Geometry: see drawing. Coordinates: mm, zero at the bounding-box minimum. A direction names the side the tool comes from. Give positions to 0.01 mm unless a question says otherwise; leave off trailing zeros. Order: outer loops, then holes, each group sorted by start corner. A loop starts at its lowest first (then second) coordinate and runs counter-clockwise, first axis right, second up. Notation, with made-up numbers: (82, 51) - (137, 51) arc R30 ccw to (137, 84) - close; hole circle Ø2 at (31.25, -20.5). An arc over 180 degrees is marked (long way). Write item = value, one per line. Start each with the question number.
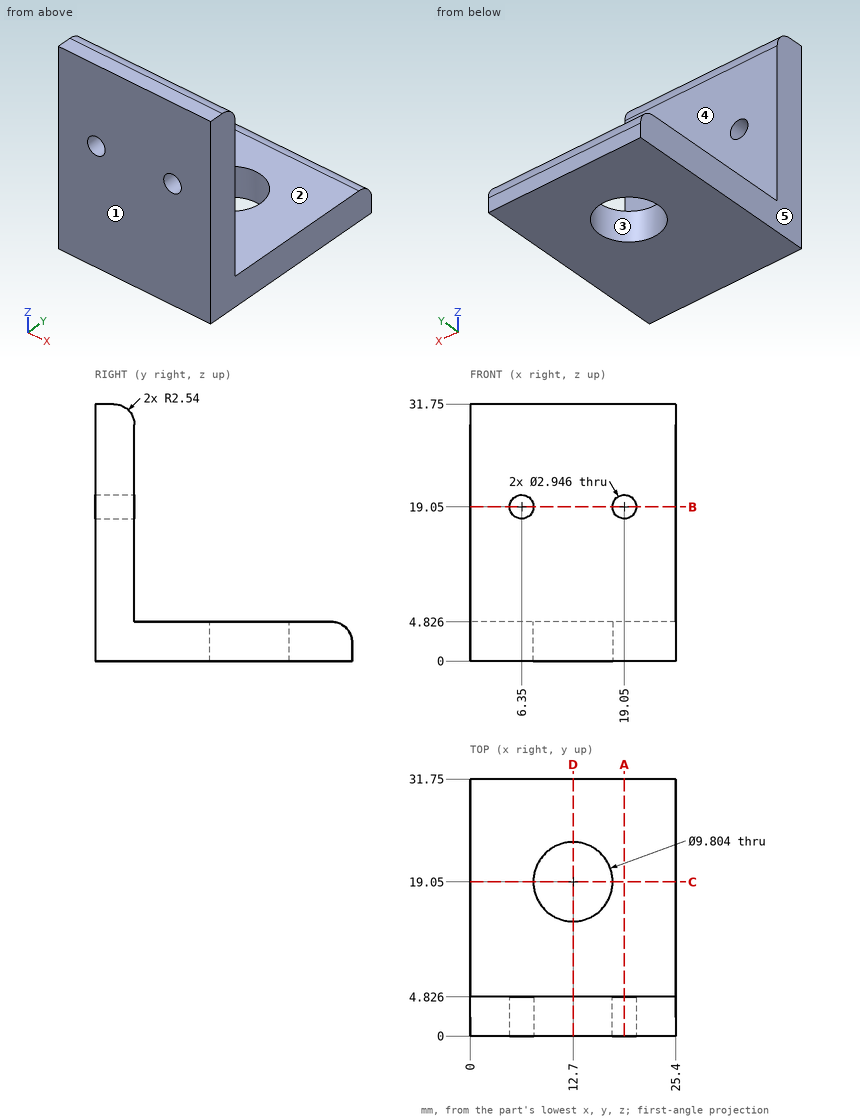
Q1. Material intervals for line 1 along X through (y, z) = (3.3, 19.05); line 2 along X through (y, z) = (19, 2); line 3 along Z through (x, y) = (6.35, 2.4), sorted ascending. Write a range as from..to.
Q2. Contact query for a flat-ended pin moving along its axis: pin 1 (8 mm diameter, centred on x = 19.5, y = 14, fed in from +Z). Output: stop coordinate, or through.
Q3. Pull-direction query (Y, two-part tool) for the marked faces 3, 4 and 5; classes: +Y half, -Y half, draft (parallel to the pull), parting line (faces both ways), or undercut.
Q4. Section B-B, the plane z = 19.05. Return the cut outline in (x, y).
Q5. Section A-A, the plane x = 19.05. Return the cut outline in (y, z), then the cut area to 3 significant figures.
Q6. Set-up query: the marked faces 1 and 2. Return all of +Z, -Z, +X, -X, +Y, -Y with unobstructed straight access to the full face (end or side cutting, diameter ignored); none if empty.
Q7. Section D-D, the plane x = 12.7. Return the cut outline in (y, z).
Q8. Section C-C, the plane y = 19.05. Return the cut outline in (x, z).
The answers:
q1.line_1 = 0..4.88, 7.82..17.58, 20.52..25.4
q1.line_2 = 0..7.8, 17.6..25.4
q1.line_3 = 0..17.58, 20.52..31.75
q2.pin_1 = 4.83
q3.face_3 = undercut
q3.face_4 = +Y half
q3.face_5 = draft
q4.outline = (0, 0) - (4.88, 0) - (4.88, 4.83) - (0, 4.83) - close; (7.82, 0) - (17.58, 0) - (17.58, 4.83) - (7.82, 4.83) - close; (20.52, 0) - (25.4, 0) - (25.4, 4.83) - (20.52, 4.83) - close
q5.outline = (0, 0) - (31.75, 0) - (31.75, 2.29) arc R2.54 ccw to (29.21, 4.83) - (4.83, 4.83) - (4.83, 17.58) - (0, 17.58) - close; (0, 20.52) - (4.83, 20.52) - (4.83, 29.21) arc R2.54 ccw to (2.29, 31.75) - (0, 31.75) - close
q5.area = 266 mm²
q6.face_1 = +Z, -Z, +X, -X, -Y
q6.face_2 = +Z, +X, -X, +Y
q7.outline = (0, 0) - (14.15, 0) - (14.15, 4.83) - (4.83, 4.83) - (4.83, 29.21) arc R2.54 ccw to (2.29, 31.75) - (0, 31.75) - close; (23.95, 0) - (31.75, 0) - (31.75, 2.29) arc R2.54 ccw to (29.21, 4.83) - (23.95, 4.83) - close
q8.outline = (0, 0) - (7.8, 0) - (7.8, 4.83) - (0, 4.83) - close; (17.6, 0) - (25.4, 0) - (25.4, 4.83) - (17.6, 4.83) - close
